Check sheet for the modelled part. Datum: model origin and axes. Units: mm. Give positions to 0.01 mm unless a question says otherwise; leave off trailing zeros. Order: outer loops, then holes, each group sorted by start corner. A loop starts at its lowest first (then second) coordinate and runs counter-clockwise, first axis right, second up.
Item 1: Release check for a two-part mould opening along X. For faces 1 (the flat face through (93, 27, 1)), 2 (the flat face through (-93, 32, -1)), 3 (the flat face through (22, 30, 91)), 4 (the flat face through (-69, 5, 22)) record: released by +X, released by -X, zero draft, split by the parting line, or undercut.
Item 2: Sectioned sample at B-B on z = -8. Record the boundary of the cut face in (x, y).
Item 3: Sectioned sample at A-A on x = -19.5. Record the boundary of the cut face in (y, z), and give its area (3 significant figures).
Item 4: Gauge pin test, flat ends, axial feed: P1, Ø12.5, axis at x = -63.5, y = 56.5, coming from the +Z side; P2, Ø6, axis at x = -60, z = -76.5, coming from the +Y side. Record the tip position at first contact, or that the pin passes through.
Item 5: Material ranges on line 1 along Z through (x, y) = (-35, 47); line 2 along X through (y, z) = (71, -55.5), recorded low to high.
Item 6: Sectioned sample at C-C on y = 63.5. Count the separate pieces of the cut face and the enclosed holes in it, and give its area (3 significant figures).
from build123d import *

# Parameters (mm, degrees)
SKETCH1_W                   = 186
SKETCH1_H                   = 186
BOSS_EXTRUDE1_DEPTH         = 5
SKETCH2_W                   = 23
SKETCH2_H                   = 24
SKETCH2_W_2                 = 20
SKETCH2_H_2                 = 20
BOSS_EXTRUDE2_DEPTH         = 80
LPATTERN1_COUNT             = 2
LPATTERN1_PITCH             = 22
MIRROR1_COPY_1_SKETCH_W     = 23
MIRROR1_COPY_1_SKETCH_H     = 24
MIRROR1_COPY_1_SKETCH_W_2   = 20
MIRROR1_COPY_1_SKETCH_H_2   = 20
MIRROR1_COPY_1_DEPTH        = 80
SKETCH3_W                   = 1
SKETCH3_H                   = 48
BOSS_EXTRUDE3_DEPTH         = 80
SKETCH4_W                   = 48
SKETCH4_H                   = 48
SKETCH4_W_2                 = 44
SKETCH4_H_2                 = 44
BOSS_EXTRUDE4_DEPTH         = 50
LPATTERN2_COUNT             = 3
LPATTERN2_PITCH             = 46
LPATTERN3_COUNT             = 4
LPATTERN3_PITCH             = 46
LPATTERN3_COPY_1_SKETCH_W   = 48
LPATTERN3_COPY_1_SKETCH_H   = 48
LPATTERN3_COPY_1_SKETCH_W_2 = 44
LPATTERN3_COPY_1_SKETCH_H_2 = 44
LPATTERN3_COPY_1_DEPTH      = 50
LPATTERN3_COPY_2_SKETCH_W   = 48
LPATTERN3_COPY_2_SKETCH_H   = 48
LPATTERN3_COPY_2_SKETCH_W_2 = 44
LPATTERN3_COPY_2_SKETCH_H_2 = 44
LPATTERN3_COPY_2_DEPTH      = 50
LPATTERN3_COPY_3_SKETCH_W   = 48
LPATTERN3_COPY_3_SKETCH_H   = 48
LPATTERN3_COPY_3_SKETCH_W_2 = 44
LPATTERN3_COPY_3_SKETCH_H_2 = 44
LPATTERN3_COPY_3_DEPTH      = 50
LPATTERN3_COPY_4_SKETCH_W   = 48
LPATTERN3_COPY_4_SKETCH_H   = 48
LPATTERN3_COPY_4_SKETCH_W_2 = 44
LPATTERN3_COPY_4_SKETCH_H_2 = 44
LPATTERN3_COPY_4_DEPTH      = 50
LPATTERN3_COPY_5_SKETCH_W   = 48
LPATTERN3_COPY_5_SKETCH_H   = 48
LPATTERN3_COPY_5_SKETCH_W_2 = 44
LPATTERN3_COPY_5_SKETCH_H_2 = 44
LPATTERN3_COPY_5_DEPTH      = 50
LPATTERN3_COPY_6_SKETCH_W   = 48
LPATTERN3_COPY_6_SKETCH_H   = 48
LPATTERN3_COPY_6_SKETCH_W_2 = 44
LPATTERN3_COPY_6_SKETCH_H_2 = 44
LPATTERN3_COPY_6_DEPTH      = 50
BOSS_EXTRUDE6_DEPTH         = 50
SKETCH9_W                   = 136
SKETCH9_H                   = 136
CUT_EXTRUDE2_DEPTH          = 50
FILLET1_R                   = 2
FILLET2_R                   = 2


with BuildPart() as part:
    # Sketch1 → Boss-Extrude1 (new body)
    with BuildSketch(Plane(origin=(0, 0, 0), x_dir=(1, 0, 0), z_dir=(0, 1, 0))):
        Rectangle(SKETCH1_W, SKETCH1_H)
    extrude(amount=BOSS_EXTRUDE1_DEPTH)

    # Sketch2 → Boss-Extrude2 (add)
    with BuildSketch(Plane(origin=(0, 5, 0), x_dir=(1, 0, 0), z_dir=(0, 1, 0))):
        with Locations((-81.5, 81)):
            Rectangle(SKETCH2_W, SKETCH2_H)
        with Locations((-81, 81)):
            Rectangle(SKETCH2_W_2, SKETCH2_H_2, mode=Mode.SUBTRACT)
    boss_extrude2 = extrude(amount=BOSS_EXTRUDE2_DEPTH)

    # LPattern1: Boss-Extrude2 ×2
    with Locations(*[(i * LPATTERN1_PITCH, 0, 0) for i in range(1, LPATTERN1_COUNT)]):
        add(boss_extrude2)

    # Mirror1: Boss-Extrude2 across plane
    add(boss_extrude2.mirror(Plane(origin=(-93, 85, -69), x_dir=(1, 0, 0), z_dir=(0, 0, -1))))

    # Mirror1 copy 1 sketch → Mirror1 copy 1 (add)
    with BuildSketch(Plane(origin=(22, 5, -138), x_dir=(1, 0, 0), z_dir=(0, 1, 0))):
        with Locations((-81.5, -81)):
            Rectangle(MIRROR1_COPY_1_SKETCH_W, MIRROR1_COPY_1_SKETCH_H)
        with Locations((-81, -81)):
            Rectangle(MIRROR1_COPY_1_SKETCH_W_2, MIRROR1_COPY_1_SKETCH_H_2, mode=Mode.SUBTRACT)
    extrude(amount=MIRROR1_COPY_1_DEPTH)

    # Sketch3 → Boss-Extrude3 (add)
    with BuildSketch(Plane(origin=(0, 5, 0), x_dir=(1, 0, 0), z_dir=(0, 1, 0))):
        with Locations((-47.5, 69)):
            Rectangle(SKETCH3_W, SKETCH3_H)
    extrude(amount=BOSS_EXTRUDE3_DEPTH)

    # Sketch4 → Boss-Extrude4 (add)
    with BuildSketch(Plane(origin=(0, 5, 0), x_dir=(1, 0, 0), z_dir=(0, 1, 0))):
        with Locations((-23, 69)):
            Rectangle(SKETCH4_W, SKETCH4_H)
        with Locations((-23, 69)):
            Rectangle(SKETCH4_W_2, SKETCH4_H_2, mode=Mode.SUBTRACT)
    boss_extrude4 = extrude(amount=BOSS_EXTRUDE4_DEPTH)

    # LPattern2: Boss-Extrude4 ×3
    with Locations(*[(i * LPATTERN2_PITCH, 0, 0) for i in range(1, LPATTERN2_COUNT)]):
        add(boss_extrude4)

    # LPattern3: Boss-Extrude4 ×4
    with Locations(*[(0, 0, i * LPATTERN3_PITCH) for i in range(1, LPATTERN3_COUNT)]):
        add(boss_extrude4)

    # LPattern3 copy 1 sketch → LPattern3 copy 1 (add)
    with BuildSketch(Plane(origin=(46, 5, 46), x_dir=(1, 0, 0), z_dir=(0, 1, 0))):
        with Locations((-23, 69)):
            Rectangle(LPATTERN3_COPY_1_SKETCH_W, LPATTERN3_COPY_1_SKETCH_H)
        with Locations((-23, 69)):
            Rectangle(LPATTERN3_COPY_1_SKETCH_W_2, LPATTERN3_COPY_1_SKETCH_H_2, mode=Mode.SUBTRACT)
    extrude(amount=LPATTERN3_COPY_1_DEPTH)

    # LPattern3 copy 2 sketch → LPattern3 copy 2 (add)
    with BuildSketch(Plane(origin=(46, 5, 92), x_dir=(1, 0, 0), z_dir=(0, 1, 0))):
        with Locations((-23, 69)):
            Rectangle(LPATTERN3_COPY_2_SKETCH_W, LPATTERN3_COPY_2_SKETCH_H)
        with Locations((-23, 69)):
            Rectangle(LPATTERN3_COPY_2_SKETCH_W_2, LPATTERN3_COPY_2_SKETCH_H_2, mode=Mode.SUBTRACT)
    extrude(amount=LPATTERN3_COPY_2_DEPTH)

    # LPattern3 copy 3 sketch → LPattern3 copy 3 (add)
    with BuildSketch(Plane(origin=(46, 5, 138), x_dir=(1, 0, 0), z_dir=(0, 1, 0))):
        with Locations((-23, 69)):
            Rectangle(LPATTERN3_COPY_3_SKETCH_W, LPATTERN3_COPY_3_SKETCH_H)
        with Locations((-23, 69)):
            Rectangle(LPATTERN3_COPY_3_SKETCH_W_2, LPATTERN3_COPY_3_SKETCH_H_2, mode=Mode.SUBTRACT)
    extrude(amount=LPATTERN3_COPY_3_DEPTH)

    # LPattern3 copy 4 sketch → LPattern3 copy 4 (add)
    with BuildSketch(Plane(origin=(92, 5, 46), x_dir=(1, 0, 0), z_dir=(0, 1, 0))):
        with Locations((-23, 69)):
            Rectangle(LPATTERN3_COPY_4_SKETCH_W, LPATTERN3_COPY_4_SKETCH_H)
        with Locations((-23, 69)):
            Rectangle(LPATTERN3_COPY_4_SKETCH_W_2, LPATTERN3_COPY_4_SKETCH_H_2, mode=Mode.SUBTRACT)
    extrude(amount=LPATTERN3_COPY_4_DEPTH)

    # LPattern3 copy 5 sketch → LPattern3 copy 5 (add)
    with BuildSketch(Plane(origin=(92, 5, 92), x_dir=(1, 0, 0), z_dir=(0, 1, 0))):
        with Locations((-23, 69)):
            Rectangle(LPATTERN3_COPY_5_SKETCH_W, LPATTERN3_COPY_5_SKETCH_H)
        with Locations((-23, 69)):
            Rectangle(LPATTERN3_COPY_5_SKETCH_W_2, LPATTERN3_COPY_5_SKETCH_H_2, mode=Mode.SUBTRACT)
    extrude(amount=LPATTERN3_COPY_5_DEPTH)

    # LPattern3 copy 6 sketch → LPattern3 copy 6 (add)
    with BuildSketch(Plane(origin=(92, 5, 138), x_dir=(1, 0, 0), z_dir=(0, 1, 0))):
        with Locations((-23, 69)):
            Rectangle(LPATTERN3_COPY_6_SKETCH_W, LPATTERN3_COPY_6_SKETCH_H)
        with Locations((-23, 69)):
            Rectangle(LPATTERN3_COPY_6_SKETCH_W_2, LPATTERN3_COPY_6_SKETCH_H_2, mode=Mode.SUBTRACT)
    extrude(amount=LPATTERN3_COPY_6_DEPTH)

    # Sketch6 → Boss-Extrude6 (add)
    with BuildSketch(Plane(origin=(0, 5, 0), x_dir=(1, 0, 0), z_dir=(0, 1, 0))):
        Polygon((-47, -93), (-47, -91), (-91, -91), (-91, 45), (-93, 45), (-93, -93), align=None)
    extrude(amount=BOSS_EXTRUDE6_DEPTH)

    # Sketch9 → Cut-Extrude2 (cut)
    with BuildSketch(Plane(origin=(0, 5, 0), x_dir=(1, 0, 0), z_dir=(0, 1, 0))):
        with Locations((23, -23)):
            Rectangle(SKETCH9_W, SKETCH9_H)
    extrude(amount=CUT_EXTRUDE2_DEPTH, mode=Mode.SUBTRACT)

    # Fillet1
    fillet1_edges = [part.edges().sort_by_distance(p)[0] for p in [
        (-69, 45, -47),
        (-49, 45, -47),
        (-49, 45, -67),
        (-69, 45, -67),
        (-47, 70, -93),
        (-45, 30, -91),
        (-45, 30, -47),
        (-1, 30, -47),
        (-1, 30, -91),
        (47, 30, -47),
        (1, 30, -91),
        (1, 30, -47),
        (45, 30, -47),
        (45, 30, -91),
        (47, 30, -91),
        (91, 30, -47),
        (91, 30, -91),
        (-91, 45, -71),
        (-71, 45, -71),
        (-71, 45, -91),
        (-91, 45, -91),
        (-47, 30, -45),
        (-45, 30, -45),
        (-45, 30, 91),
        (91, 30, -45),
        (91, 30, 91),
        (-47, 30, 91),
        (-91, 30, 91),
        (-91, 30, -45),
        (-69, 45, -71),
        (-49, 45, -71),
        (-49, 45, -91),
        (-69, 45, -91),
        (-93, 42.5, -93),
        (93, 27.5, -93),
        (93, 27.5, 93),
        (-93, 27.5, 93),
        (-91, 45, -47),
        (-71, 45, -47),
    ]]
    fillet(fillet1_edges, radius=FILLET1_R)

    # Fillet2
    fillet2_edges = [part.edges().sort_by_distance(p)[0] for p in [
        (-47, 70, -45),
        (-93, 70, -45),
    ]]
    fillet(fillet2_edges, radius=FILLET2_R)


solid = part.part
Report:
1. face 1: released by +X
1. face 2: released by -X
1. face 3: undercut
1. face 4: undercut
2. outline: (-93, 0) - (93, 0) - (93, 55) - (91, 55) - (91, 5) - (-45, 5) - (-45, 55) - (-47, 55) - (-47, 5) - (-91, 5) - (-91, 55) - (-93, 55) - close
3. outline: (0, -93) - (55, -93) - (55, -91) - (5, -91) - (5, -47) - (55, -47) - (55, -45) - (5, -45) - (5, 91) - (55, 91) - (55, 93) - (0, 93) - close
3. area: 1,230 mm2
4. P1: stops at z = 93
4. P2: stops at y = 5
5. line 1: z = -93 to -91, -47 to -45, 91 to 93
5. line 2: x = -93 to -91, -71 to -69, -49 to -47
6. separate pieces: 1
6. enclosed holes: 4
6. area: 617 mm2
